Build history of the part. All positions in model axes, mm. Give positions to 0.01 mm unless a question says otherwise; leave off trailing zeros. Put each result on its own line as item: value.
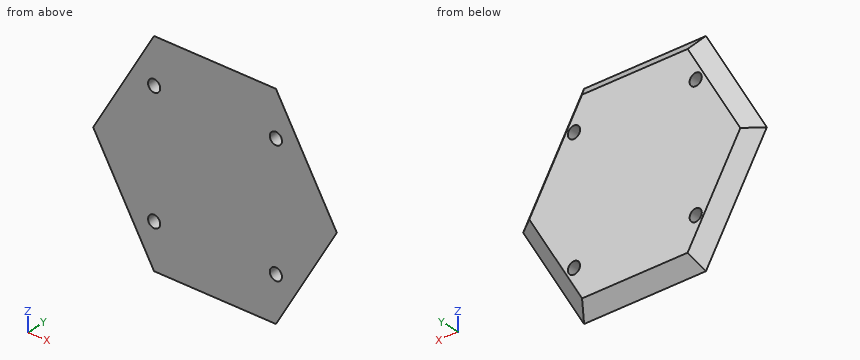
```python
from build123d import *

# Parameters (mm, degrees)
SKETCH4_R          = 2.5
CUT_EXTRUDE1_DEPTH = 5
SKETCH5_R          = 2.5
CUT_EXTRUDE2_DEPTH = 5
SKETCH6_R          = 2.5
CUT_EXTRUDE3_DEPTH = 5
SKETCH7_R          = 2.5
CUT_EXTRUDE4_DEPTH = 5


with BuildPart() as part:
    # Sketch1 → Loft3 section 0
    with BuildSketch(Plane(origin=(0, 0, 0), x_dir=(1, 0, 0), z_dir=(0, 1, 0))):
        with BuildLine():
            Line((50.051560618, 0), (25.025780309, 43.345922995))
            Line((25.025780309, 43.345922995), (-25.025780309, 43.345922995))
            Line((-25.025780309, 43.345922995), (-50.051560618, 0))
            Line((-50.051560618, 0), (-25.025780309, -43.345922995))
            Line((-25.025780309, -43.345922995), (25.025780309, -43.345922995))
            Line((25.025780309, -43.345922995), (50.051560618, 0))
        make_face()
    # Sketch2 → Loft3 section 1
    with BuildSketch(Plane(origin=(0, 5, 0), x_dir=(1, 0, 0), z_dir=(0, 1, 0))):
        with BuildLine():
            Line((43.345922995, 0), (21.672961497, 37.538670464))
            Line((21.672961497, 37.538670464), (-21.672961497, 37.538670464))
            Line((-21.672961497, 37.538670464), (-43.345922995, 0))
            Line((-43.345922995, 0), (-21.672961497, -37.538670464))
            Line((-21.672961497, -37.538670464), (21.672961497, -37.538670464))
            Line((21.672961497, -37.538670464), (43.345922995, 0))
        make_face()
    loft()

    # Sketch4 → Cut-Extrude1 (cut)
    with BuildSketch(Plane(origin=(0, 5, 0), x_dir=(1, 0, 0), z_dir=(0, 1, 0))):
        with Locations(Location((-25, 25, 0), (0, 0, 270))):
            Circle(SKETCH4_R)
    extrude(amount=-CUT_EXTRUDE1_DEPTH, mode=Mode.SUBTRACT)

    # Sketch5 → Cut-Extrude2 (cut)
    with BuildSketch(Plane(origin=(0, 5, 0), x_dir=(1, 0, 0), z_dir=(0, 1, 0))):
        with Locations(Location((25, 25, 0), (0, 0, 270))):
            Circle(SKETCH5_R)
    extrude(amount=-CUT_EXTRUDE2_DEPTH, mode=Mode.SUBTRACT)

    # Sketch6 → Cut-Extrude3 (cut)
    with BuildSketch(Plane(origin=(0, 5, 0), x_dir=(1, 0, 0), z_dir=(0, 1, 0))):
        with Locations(Location((-25, -25, 0), (0, 0, 270))):
            Circle(SKETCH6_R)
    extrude(amount=-CUT_EXTRUDE3_DEPTH, mode=Mode.SUBTRACT)

    # Sketch7 → Cut-Extrude4 (cut)
    with BuildSketch(Plane(origin=(0, 5, 0), x_dir=(1, 0, 0), z_dir=(0, 1, 0))):
        with Locations(Location((25, -25, 0), (0, 0, 270))):
            Circle(SKETCH7_R)
    extrude(amount=-CUT_EXTRUDE4_DEPTH, mode=Mode.SUBTRACT)


solid = part.part
```
Q1. Slice it at A-A (y = 4). State how many separate pieces and enclosed holes the cut face has, and give its area (3 significant figures).
Here are the results:
separate pieces: 1
enclosed holes: 4
area: 5,110 mm²
Q2. Probe line 1 (X direction, y = 3.9, z = -25); line 2 (X direction, y = 3.6, z = -23.5); line 3 (Z direction, x = -4, y = 3.3). List the from-to ranges inside material, lowest first. Write a range as from..to.
Here are the results:
line 1: -30.39..-27.5, -22.5..22.5, 27.5..30.39
line 2: -31.66..-27, -23..23, 27..31.66
line 3: -39.51..39.51
Q3. Drop flat-ended pins along their axis: pin 1 Ø4 at (x, z) = (25, 25) entering from -Y; pin 2 Ø1 at (x, z) = (-20.5, 8) entering from -Y; pin 3 Ø1 at (y, z) = (3.5, 10) entering from +X; pin 4 Ø1.5 at (x, y) = (-2, 1.5) entering from -Z. Give the stop position or say it passes through.
Here are the results:
pin 1: through
pin 2: y = 0
pin 3: x = 40.31
pin 4: z = -42.47
